```python
from build123d import *

# Parameters (mm, degrees)
F0_W     = 71
F0_H     = 58
F1_DEPTH = 1.5
F3_R     = 1.778
F4_DEPTH = 25
F6_DEPTH = 71.001
F7_R     = 3


with BuildPart() as f1:
    # F0 (on Top) → F1 (new body)
    with BuildSketch(Plane.XY):
        Rectangle(F0_W, F0_H)
    extrude(amount=F1_DEPTH)

    # F3 (on face) → F4 (join)
    with BuildSketch(Plane.XY.offset(1.5)):
        Polygon((35.5, -29), (35.5, 29), (-31.925, 29), (-35.5, 29), (-35.5, 23.9875), (-35.5, -29), align=None)
        with Locations((-31.182, -24.682)):
            Circle(F3_R, mode=Mode.SUBTRACT)
        with Locations((31.182, -24.682)):
            Circle(F3_R, mode=Mode.SUBTRACT)
        with Locations((-31.182, 24.682)):
            Circle(F3_R, mode=Mode.SUBTRACT)
        with BuildLine():
            Line((-26.864, 27.5), (26.864, 27.5))
            Line((26.864, 27.5), (26.864, 24.682))
            ThreePointArc((26.864, 24.682), (28.1287129188, 21.6287129188), (31.182, 20.364))
            Line((31.182, 20.364), (34, 20.364))
            Line((34, 20.364), (34, -20.364))
            Line((34, -20.364), (31.182, -20.364))
            ThreePointArc((31.182, -20.364), (28.1287129188, -21.6287129188), (26.864, -24.682))
            Line((26.864, -24.682), (26.864, -27.5))
            Line((26.864, -27.5), (-26.864, -27.5))
            Line((-26.864, -27.5), (-26.864, -24.682))
            ThreePointArc((-26.864, -24.682), (-28.1287129188, -21.6287129188), (-31.182, -20.364))
            Line((-31.182, -20.364), (-34, -20.364))
            Line((-34, -20.364), (-34, 20.364))
            Line((-34, 20.364), (-31.182, 20.364))
            ThreePointArc((-31.182, 20.364), (-28.1287129188, 21.6287129188), (-26.864, 24.682))
            Line((-26.864, 24.682), (-26.864, 27.5))
        make_face(mode=Mode.SUBTRACT)
        with Locations((31.182, 24.682)):
            Circle(F3_R, mode=Mode.SUBTRACT)
    extrude(amount=F4_DEPTH)

    # F5 (on face) → F6 (cut, through all)
    with BuildSketch(Plane.YZ.offset(35.5)):
        with BuildLine():
            Line((-8.60102, 26.5), (-8.60102, 16.5))
            ThreePointArc((-8.60102, 16.5), (-1.60102, 9.5), (5.39898, 16.5))
            Line((5.39898, 16.5), (5.39898, 26.5))
            Line((5.39898, 26.5), (-8.60102, 26.5))
        make_face()
    extrude(amount=-F6_DEPTH, mode=Mode.SUBTRACT)

    # F7
    f7_edges = [f1.edges().sort_by_distance(p)[0] for p in [
        (35.5, 29, 13.25),
        (35.5, -29, 13.25),
        (-35.5, 29, 13.25),
        (-35.5, -29, 13.25),
    ]]
    fillet(f7_edges, radius=F7_R)


solid = f1.part
```
Work out the finished part from the listing and answer in its coordinate system (mm). A direction names the side the tool comes from. Round coordinates to 2 decimals unless told otherwise and drop trailing zeros. Write each loop counter-clockwise with the first axis right and the second up, starting at its lowest first coordinate (ties: lowest second). Pieces come first, ordered by that corner, then holes. Notation, with made-up numbers: (28.5, 12) - (63.5, 12) arc R13 cw to (63.5, 37) - close; hole circle Ø6 at (56.25, -12.75). An arc over 180 degrees is marked (long way). Return JSON: item names as keys, results as strings. Group by question number.
Q1. The part is cut by section D-D on y = 16. Write down the section's boundary in (x, z), then the cut area to 4 significant figures.
Q2. Find the intervals of material crossed by L1, parallel to X at y = 6, z = 20.5; L2, parallel to Y at x = -2.5, z = 18.5; L3, parallel to X at y = -24.5, z = 3.5, in increasing order.
Q3. The part is cut by section B-B on x = -12. Write down the section's boundary in (y, z).
Q4. The mould has two halves that part along X. Classify faces 3 (the flat face through (0, 0, 1.5)), 4 (the flat face through (0, 29, 13)), 5 (the cylindrical face through (-34.6, 28.14, 13.44)): released by +X, released by -X, zero draft, split by the parting line, or undercut.
Q5. This flat-tipped pin is pushed along its axis until it touches: pin 1 Ø1.1 at (x, y) = (30.5, 24) entering from +Z. Where does it stop, or does it pass through?
Q6. The part is cut by section C-C on z = 18.75. Count the separate pieces of the cut face and the enclosed holes in it, then the cut area to 3 significant figures.
Q7. The part is cut by section A-A on z = 6. Write down the section's boundary in (x, y).
Q8. For faces 1 (the cylindrical face through (-34.74, -1.75, 9.5)), 2 (the flat face through (-33, -20.364, 14)), determine the directions among +Z, -Z, +X, -X, +Y, -Y from which every point of the face is accessible in a straight line to the end or side of a thin tool.
Solved:
{
 "1": {"outline": "(-35.5, 0) - (35.5, 0) - (35.5, 26.5) - (34, 26.5) - (34, 1.5) - (-34, 1.5) - (-34, 26.5) - (-35.5, 26.5) - close", "area": "181.5 mm²"},
 "2": {"L1": "-35.5 to -34, 34 to 35.5", "L2": "-29 to -27.5, 27.5 to 29", "L3": "-35.5 to -32.95, -29.41 to -26.87, 26.87 to 29.41, 32.95 to 35.5"},
 "3": {"outline": "(-29, 0) - (29, 0) - (29, 26.5) - (27.5, 26.5) - (27.5, 1.5) - (-27.5, 1.5) - (-27.5, 26.5) - (-29, 26.5) - close"},
 "4": {"face 3": "undercut", "face 4": "zero draft", "face 5": "released by -X"},
 "5": {"pin 1": "z = 1.5"},
 "6": {"separate pieces": "2", "enclosed holes": "4", "area": "476 mm²"},
 "7": {"outline": "(-35.5, -26) arc R3 ccw to (-32.5, -29) - (32.5, -29) arc R3 ccw to (35.5, -26) - (35.5, 26) arc R3 ccw to (32.5, 29) - (-32.5, 29) arc R3 ccw to (-35.5, 26) - close; hole (-34, -20.36) - (-31.18, -20.36) arc R4.32 cw to (-26.86, -24.68) - (-26.86, -27.5) - (26.86, -27.5) - (26.86, -24.68) arc R4.32 cw to (31.18, -20.36) - (34, -20.36) - (34, 20.36) - (31.18, 20.36) arc R4.32 cw to (26.86, 24.68) - (26.86, 27.5) - (-26.86, 27.5) - (-26.86, 24.68) arc R4.32 cw to (-31.18, 20.36) - (-34, 20.36) - close; hole circle Ø3.56 at (-31.18, -24.68); hole circle Ø3.56 at (-31.18, 24.68); hole circle Ø3.56 at (31.18, -24.68); hole circle Ø3.56 at (31.18, 24.68)"},
 "8": {"face 1": "+Z, +X, -X", "face 2": "+Z"}
}
